Source: CAD feature listing. Evaluate the final solid. Frame: model axes, mm. Round coordinates to 2 decimals unless told otherwise and drop trailing zeros. Loops run counter-clockwise (first coordinate to the right, second up) from the corner with the lowest first, then second, coordinate; pieces in that order, holes last.
(1) First-contact query: pin 1 Ø8 at (x, y) = (-8, -16) entering from -Z; pin 2 Ø0.8 at (x, z) = (25.5, 0.5) entering from +Y; pin 3 Ø0.5 at (x, z) = (25, 0.5) entering from -Y. Flat tips, straight axial feed; report the tip coordinate or a pass-through.
(2) Section B-B, the plane y = -1.5. Return the cut outline in (x, z), plus the area to 3 significant figures.
(3) Material intervals for probe 1 along Y at (x, z) = (25, 0.85); probe 2 along X at (y, z) = (1, 1.2); probe 3 along Y at (x, z) = (-10.5, 0.35), sorted ascending.
(4) Section A-A, the plane y = 15. Return the cut outline in (x, z).
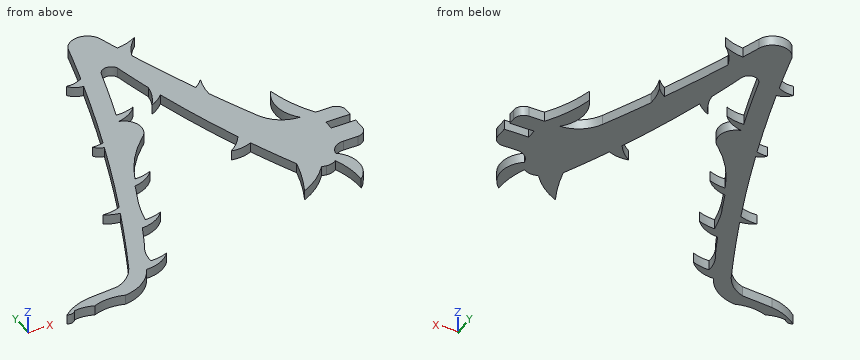
```python
from build123d import *

# Parameters (mm, degrees)
BOSS_EXTRUDE1_DEPTH = 1.524


with BuildPart() as part:
    # Sketch1 → Boss-Extrude1 (new body)
    with BuildSketch(Plane.XY):
        with BuildLine():
            Line((23.841868496, -10.506949106), (26.068199276, -10.505871764))
            ThreePointArc((26.068199276, -10.505871764), (27.147715357, -10.058146709), (27.594179967, -8.978108726))
            Line((27.594179967, -8.978108726), (27.592193648, -7.149905424))
            Line((27.592193648, -7.149905424), (23.848771017, -7.149905424))
            Line((23.848771017, -7.149905424), (23.846783681, -5.623924224))
            Line((23.846783681, -5.623924224), (27.590206312, -5.623924224))
            Line((27.590206312, -5.623924224), (27.592193648, -4.513216426))
            ThreePointArc((27.592193648, -4.513216426), (27.145243923, -3.434184592), (26.06621194, -2.987235226))
            Line((26.06621194, -2.987235226), (23.700742448, -2.987731933))
            ThreePointArc((23.700742448, -2.987731933), (21.853763211, 0.396085968), (20.662942507, 4.062624108))
            ThreePointArc((20.662942507, 4.062624108), (19.722128306, 0.415432016), (21.335272956, -2.98822864))
            ThreePointArc((21.335272956, -2.98822864), (18.47901593, -2.097405096), (16.50646059, 0.152216254))
            ThreePointArc((16.50646059, 0.152216254), (14.785372428, 3.836585951), (13.130721746, 7.551267048))
            ThreePointArc((13.130721746, 7.551267048), (13.233622121, 9.252516805), (13.653748602, 10.904283424))
            ThreePointArc((13.653748602, 10.904283424), (12.99040582, 10.220702416), (12.234885694, 9.64061968))
            ThreePointArc((12.234885694, 9.64061968), (10.12080113, 14.817724102), (8.135197678, 20.045452354))
            ThreePointArc((8.135197678, 20.045452354), (9.07398957, 21.945137091), (10.469509483, 23.539708032))
            ThreePointArc((10.469509483, 23.539708032), (8.915709374, 22.846825686), (7.245789765, 22.521634627))
            ThreePointArc((7.245789765, 22.521634627), (6.75481808, 23.928653676), (6.273116214, 25.338873202))
            ThreePointArc((6.273116214, 25.338873202), (3.955147053, 27.136861073), (1.395527385, 25.703651887))
            ThreePointArc((1.395527385, 25.703651887), (0.515712233, 22.228862241), (-0.41145202, 18.766405854))
            ThreePointArc((-0.41145202, 18.766405854), (-1.622932108, 18.279372053), (-2.926572326, 18.205832225))
            ThreePointArc((-2.926572326, 18.205832225), (-2.022011476, 17.428802856), (-0.877304936, 17.094659314))
            ThreePointArc((-0.877304936, 17.094659314), (-2.723720739, 10.849649399), (-4.724433819, 4.652347782))
            ThreePointArc((-4.724433819, 4.652347782), (-5.553363062, 4.507568674), (-6.394830907, 4.511636389))
            ThreePointArc((-6.394830907, 4.511636389), (-5.816780919, 3.946754251), (-5.053213137, 3.681805461))
            ThreePointArc((-5.053213137, 3.681805461), (-7.342468518, -2.757262031), (-9.798511581, -9.134575953))
            ThreePointArc((-9.798511581, -9.134575953), (-11.146241899, -9.494732073), (-12.539374775, -9.567328436))
            ThreePointArc((-12.539374775, -9.567328436), (-11.456387472, -10.079926299), (-10.289959872, -10.353905718))
            ThreePointArc((-10.289959872, -10.353905718), (-12.696378355, -16.085978869), (-15.23781775, -21.759478522))
            ThreePointArc((-15.23781775, -21.759478522), (-16.613838722, -23.569338635), (-18.587158788, -24.698513227))
            Line((-18.587158788, -24.698513227), (-23.337428896, -25.097915233))
            ThreePointArc((-23.337428896, -25.097915233), (-25.600837555, -25.751570827), (-27.594180508, -27.00730498))
            ThreePointArc((-27.594180508, -27.00730498), (-26.834901197, -27.111562643), (-26.224288347, -26.648392395))
            ThreePointArc((-26.224288347, -26.648392395), (-24.749884123, -26.629116362), (-23.323298678, -27.002068563))
            ThreePointArc((-23.323298678, -27.002068563), (-20.933638176, -26.512638906), (-18.521050739, -26.872417397))
            ThreePointArc((-18.521050739, -26.872417397), (-15.408520041, -25.680590506), (-13.243289855, -23.146803434))
            ThreePointArc((-13.243289855, -23.146803434), (-10.939299547, -22.644411883), (-9.09502436, -21.174916172))
            ThreePointArc((-9.09502436, -21.174916172), (-10.422629625, -21.592521303), (-11.808160337, -21.723801278))
            ThreePointArc((-11.808160337, -21.723801278), (-11.629423676, -19.87808238), (-10.869125888, -18.186759728))
            ThreePointArc((-10.869125888, -18.186759728), (-10.06288258, -16.43139287), (-9.27114661, -14.669435086))
            ThreePointArc((-9.27114661, -14.669435086), (-7.116039845, -14.110620335), (-5.392996781, -12.70069775))
            ThreePointArc((-5.392996781, -12.70069775), (-6.685933272, -13.1111928), (-8.035353311, -13.249960648))
            ThreePointArc((-8.035353311, -13.249960648), (-7.62253261, -11.397230513), (-7.080348792, -9.578146516))
            ThreePointArc((-7.080348792, -9.578146516), (-6.326640496, -7.746057309), (-5.588458433, -5.90765738))
            ThreePointArc((-5.588458433, -5.90765738), (-3.713864907, -5.272651789), (-2.213006184, -3.982397519))
            ThreePointArc((-2.213006184, -3.982397519), (-3.505942675, -4.392892568), (-4.855362713, -4.531660417))
            ThreePointArc((-4.855362713, -4.531660417), (-2.628642535, -0.376345962), (0.470998143, 3.175716628))
            ThreePointArc((0.470998143, 3.175716628), (1.472273464, 5.892268907), (-0.603369584, 7.910662945))
            ThreePointArc((-0.603369584, 7.910662945), (1.254291962, 8.549045158), (2.741948703, 9.831743755))
            ThreePointArc((2.741948703, 9.831743755), (1.32183158, 9.396106351), (-0.159629899, 9.287550016))
            ThreePointArc((-0.159629899, 9.287550016), (1.231844903, 13.808566094), (2.531714491, 18.356766568))
            ThreePointArc((2.531714491, 18.356766568), (3.762130664, 19.35895724), (5.111523048, 18.523822342))
            ThreePointArc((5.111523048, 18.523822342), (5.841359999, 15.591441368), (6.629061504, 12.674071577))
            ThreePointArc((6.629061504, 12.674071577), (6.131201427, 10.721467417), (5.150999348, 8.960861967))
            ThreePointArc((5.150999348, 8.960861967), (6.286769778, 9.611384591), (7.260885888, 10.485599644))
            ThreePointArc((7.260885888, 10.485599644), (9.421271832, 3.777976775), (11.888720554, -2.82286929))
            ThreePointArc((11.888720554, -2.82286929), (10.862715973, -4.146724537), (9.567099571, -5.208165187))
            ThreePointArc((9.567099571, -5.208165187), (11.169841142, -5.279612135), (12.712295724, -4.838342295))
            ThreePointArc((12.712295724, -4.838342295), (14.260423663, -8.421579982), (15.8996033, -11.964090751))
            ThreePointArc((15.8996033, -11.964090751), (15.065930684, -14.956168746), (13.895117254, -17.833100562))
            ThreePointArc((13.895117254, -17.833100562), (16.426590022, -16.289885632), (18.495512952, -14.166345049))
            Line((18.495512952, -14.166345049), (19.168549545, -14.30256589))
            ThreePointArc((19.168549545, -14.30256589), (20.020311576, -14.238117294), (20.784861991, -13.857177873))
            ThreePointArc((20.784861991, -13.857177873), (21.617673082, -16.43239432), (21.871894835, -19.126960215))
            ThreePointArc((21.871894835, -19.126960215), (23.381897517, -15.709462317), (21.630181539, -12.409327303))
            ThreePointArc((21.630181539, -12.409327303), (22.378657332, -11.042665903), (23.841868496, -10.506949106))
        make_face()
    extrude(amount=BOSS_EXTRUDE1_DEPTH)


solid = part.part
```
Output values:
1. pin 1: stops at z = 0
1. pin 2: stops at y = -2.99
1. pin 3: stops at y = -10.51
2. outline: (-6.88, 0) - (-3.35, 0) - (-3.35, 1.52) - (-6.88, 1.52) - close; (11.37, 0) - (17.72, 0) - (17.72, 1.52) - (11.37, 1.52) - close; (20.26, 0) - (22.79, 0) - (22.79, 1.52) - (20.26, 1.52) - close
2. area: 18.9 mm2
3. probe 1: y = -10.51 to -7.15, -5.62 to -2.99
3. probe 2: x = -5.98 to -1.59, 10.42 to 16.1, 19.7 to 21.6
3. probe 3: y = -22.41 to -21.61, -17.39 to -10.87, -10.32 to -9.36
4. outline: (-1.48, 0) - (1.58, 0) - (1.58, 1.52) - (-1.48, 1.52) - close; (6, 0) - (10.05, 0) - (10.05, 1.52) - (6, 1.52) - close
